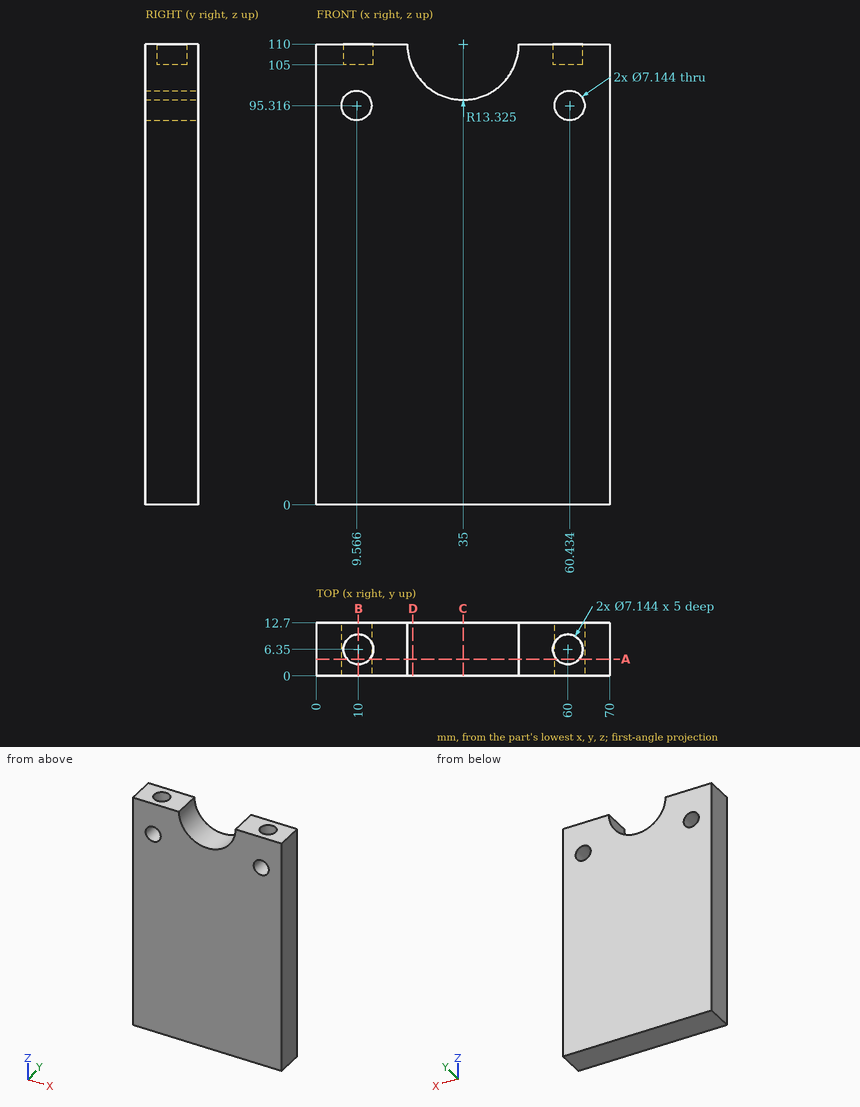
Could you check a few things on this drawing? It's one solid part, dimensions in mm from its lowest x, y, z. Coordinates: 2 decimals unless noted, no trailing zeros. Write each loop counter-clockwise with the first axis right and the second up, starting at its lowest first coordinate (ties: lowest second). Pieces come first, ordered by that corner, then holes. Notation, with made-up numbers: M 60.25,17.5 L 67.25,17.5 A26 cw 67.25,53.5 Z; hole C 86,54 d4. An arc over 180 degrees is marked long. One line per question, with ' | ' between items.
1) Imagine slicing it at C-C, the plane x = 35. Write out the boundary of the cut face in (y, z) (1 decimal).
Checks:
outline: M 0,0 L 12.7,0 L 12.7,96.7 L 0,96.7 Z
2) Imagine slicing it at D-D, the plane x = 23. Write out the boundary of the cut face in (y, z).
Checks:
outline: M 0,0 L 12.7,0 L 12.7,104.21 L 0,104.21 Z
3) Imagine slicing it at A-A, the plane y = 4. Give the number of separate pieces and of enclosed holes in the cut face, and give its area (3 significant figures).
Checks:
separate pieces: 1 | enclosed holes: 2 | area: 7,290 mm²
4) For pin 1 Ø6.5 at (x, z) = (60.43, 95.32) entering from -Y; pin 2 Ø6.5 at (x, y) = (60, 6.35) entering from +Z, each with a flat end and sliding along its axis, tell me the tip position at first contact or that it passes through.
Checks:
pin 1: through | pin 2: z = 105
5) Imagine slicing it at B-B, the plane x = 10. Write out the boundary of the cut face in (y, z), and give its area (3 significant figures).
Checks:
outline: M 0,0 L 12.7,0 L 12.7,91.77 L 0,91.77 Z; M 0,98.86 L 12.7,98.86 L 12.7,110 L 9.92,110 L 9.92,105 L 2.78,105 L 2.78,110 L 0,110 Z | area: 1,270 mm²
6) I need wall thicknesses on probe 1 along Y at (x, z) = (10, 108); probe 2 along Z at (x, y) = (60.5, 10) (1 decimal); probe 3 along X at (y, z) = (6.35, 106.1). Which ranges of each line are inside material? Lowest first, please. Write a range as [from, to].
Checks:
probe 1: [0, 2.78], [9.92, 12.7] | probe 2: [0, 91.7], [98.9, 110] | probe 3: [0, 6.43], [13.57, 22.26], [47.74, 56.43], [63.57, 70]
